The listing builds one solid part. Answer for the finished solid, in the listing's coordinates (mm). Face numbers are marked on the shaded views. Coordinates: 2 decimals unless noted, no trailing zeros. Loops run counter-clockwise (first coordinate to the right, second up) from the corner with the lowest first, then second, coordinate; pieces in that order, holes last. Notation, with made-up numbers: (32.5, 30.5) - (61.5, 30.5) arc R25 ccw to (61.5, 62.5) - close; hole circle Ø5 at (56, 33). An arc over 180 degrees is marked (long way). Write each question's results on one line, items separated by ' | '. Start each with the question number.
(1) Determine the mould class of the marked faces 1, 2 and 3 for opening direction Y: released by +Y, released by -Y, zero draft, split by the parting line, or undercut.
(2) Given pin 1 Ø1 at (x, y) = (15, -2) entering from -Z; pin 2 Ø1.4 at (x, z) = (-5.5, 0.5) entering from +Y, each flat-ended and moving along its own axis, determine where each tip first touches the part or whether it passes through.
(3) Consider line 1 (X direction, y = -3.25, z = -0.25); line 2 (Y direction, x = -4, z = 1.5); line 3 (Z direction, x = 10.5, y = 0.25). Determine where each line is inside the solid, lowest interval first. Write a range as from..to.
(4) Find section A-A on x = 9.5. Determine the outline of the cut face in (y, z) (3 decimals), then the cut area to 3 significant figures.
Autodesk Inventor part; units mm, degrees
ref_plane "Work Plane1" through (29, 0, 0) normal (0, -1, 0) x (1, 0, 0)
ref_plane "YZ Plane" through (0, 0, 0) normal (1, 0, 0) x (0, 1, 0)
ref_plane "XZ Plane" through (0, 0, 0) normal (0, 1, 0) x (-1, 0, 0)
sketch "Sketch1" plane through (0, 0, 0) normal (0, 0, 1) x (1, 0, 0)
  line L0 (-1.7145, 0) -> (38.1, 0)
  line L1 (38.1, 0) -> (38.1, 3.175)
  line L2 (38.1, 3.175) -> (12.7, 3.175)
  line L3 (12.7, 3.175) -> (10.1599, 3.175)
  line L4 (10.1599, 3.175) -> (0, 3.175)
  line L5 (0, 3.175) -> (0, 4.7625)
  line L6 (0, 4.7625) -> (-6.35, 4.7625)
  line L7 (-6.35, 4.7625) -> (-6.35, 2.7496)
  line L8 (-6.35, 2.7496) -> (-3.302, 2.7496)
  line L9 (-3.302, 2.7496) -> (-1.7145, 0)
  line L10 (-15.24, 0) -> (46.99, 0)
  line L11 (0, -0.9525) -> (0, 5.715)
  line L12 (12.7, 3.175) -> (0, 3.175) construction
  dimension "d1" = 25.4
  dimension "d2" = 2.5401
  dimension "d3" = 6.35
  dimension "d4" = 3.048
  dimension "d5" = 60
  dimension "d6" = 6.35
  dimension "d7" = 6.35
  dimension "d8" = 5.4993
  dimension "d9" = 9.525
  dimension "d26" = 38.1
revolve "Body" add sketch "Sketch1" angle 360 about axis through (-1.7145, 0, 0) along (1, 0, 0)
sketch "Sketch2" plane through (-6.35, 0, 0) normal (-1, 0, 0) x (0, 0, 1)
  circle A0 centre (0, 0) radius 2.7496
  line L0 (0, -6.6675) -> (0, 6.6675)
  line L1 (-6.6675, 0) -> (6.6675, 0)
  line L2 (2.7496, 0) -> (1.3748, -2.3812)
  line L3 (1.3748, -2.3812) -> (-1.3748, -2.3813)
  line L4 (-1.3748, -2.3813) -> (-2.7496, 0)
  line L5 (-2.7496, 0) -> (-1.3748, 2.3812)
  line L6 (-1.3748, 2.3812) -> (1.3748, 2.3813)
  line L7 (1.3748, 2.3813) -> (2.7496, 0)
extrude "Slot" add sketch "Sketch2" against normal up to next contours L7 A0 | A0 L2 | L6 L0 A0 | A0 L0 L3 | L0 L6 A0 | A0 L3 L0 | L4 A0 | A0 L5
fillet "Fillet1" radius 0.3556 1 edges at (-6.35, -4.7625, 0)
thread "Thread"
chamfer "Chamfer1" distance 0.7791 distance2 0.779 1 edges at (38.1, -3.175, 0) measured on face at (38.1, -0.6107, -1.4381)
ref_plane "Work Plane1" through (29, 0, 0) normal (0, -1, 0) x (1, 0, 0)
fillet "Fillet2" radius 0.1 1 edges at (0, -3.175, 0)
equation "\"d30\" = R"
equation "\"d17\" = RR"
equation "\"d13\" = GEL"
equation "\"d15\" = -0.5 * SPD + 0.5 * GD"
equation "\"d16\" = GUL"
equation "\"d1\" = GEL"
equation "\"d3\" = KOH"
equation "\"d4\" = INTI"
equation "\"d6\" = GD"
equation "\"d7\" = BDM"
equation "\"d8\" = 1.1547 * SW"
equation "\"d9\" = KOD"
equation "\"d26\" = NLG"
equation "\"GD\" = NND"
equation "\"NLG\" = 38.1"
equation "\"GEL\" = 25.4"
equation "\"KOD\" = 9.525"
equation "\"KOH\" = NND"
equation "\"INTI\" = 3.048"
equation "\"GAL\" = 2.54"
equation "\"GUL\" = 0.77902"
equation "\"BDM\" = NND"
equation "\"SW\" = 4.7625"
equation "\"RR\" = 0.3556"
equation "\"SPD\" = GD1"
equation "\"R\" = 0.1"
equation "\"PHH\" = 0.1 * NND"
equation "\"THREADDIA\" = 6.35"
equation "\"FAWI\" = 45deg"
equation "\"NND\" = 6.35"
equation "\"E0\" = 1.155 * SW"
equation "\"FAWI1\" = 30deg"
equation "\"TOA\" = 30deg"
equation "\"GD1\" = 4.79189"
properties part number "Unbrako - 1/4 x 1 1/2" material "Steel, Mild"
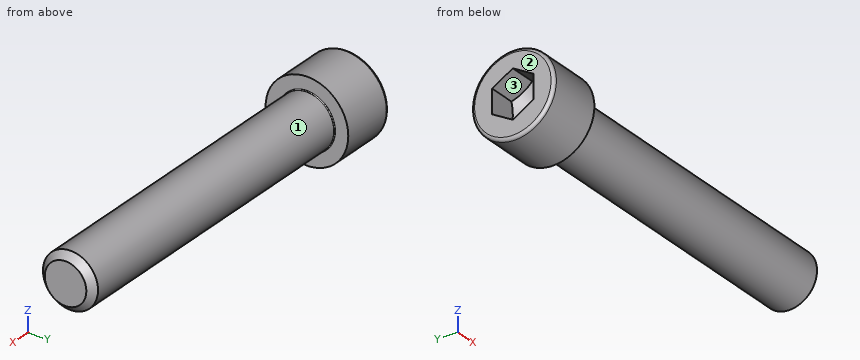
Values:
1) face 1: split by the parting line | face 2: zero draft | face 3: undercut
2) pin 1: stops at z = -2.8 | pin 2: stops at y = 4.76
3) line 1: x = -6.35..0 | line 2: y = -4.52..-2.16, 2.16..4.52 | line 3: z = -3.17..3.17
4) outline: circle Ø6.35 at (0, 0) | area: 31.7 mm²
